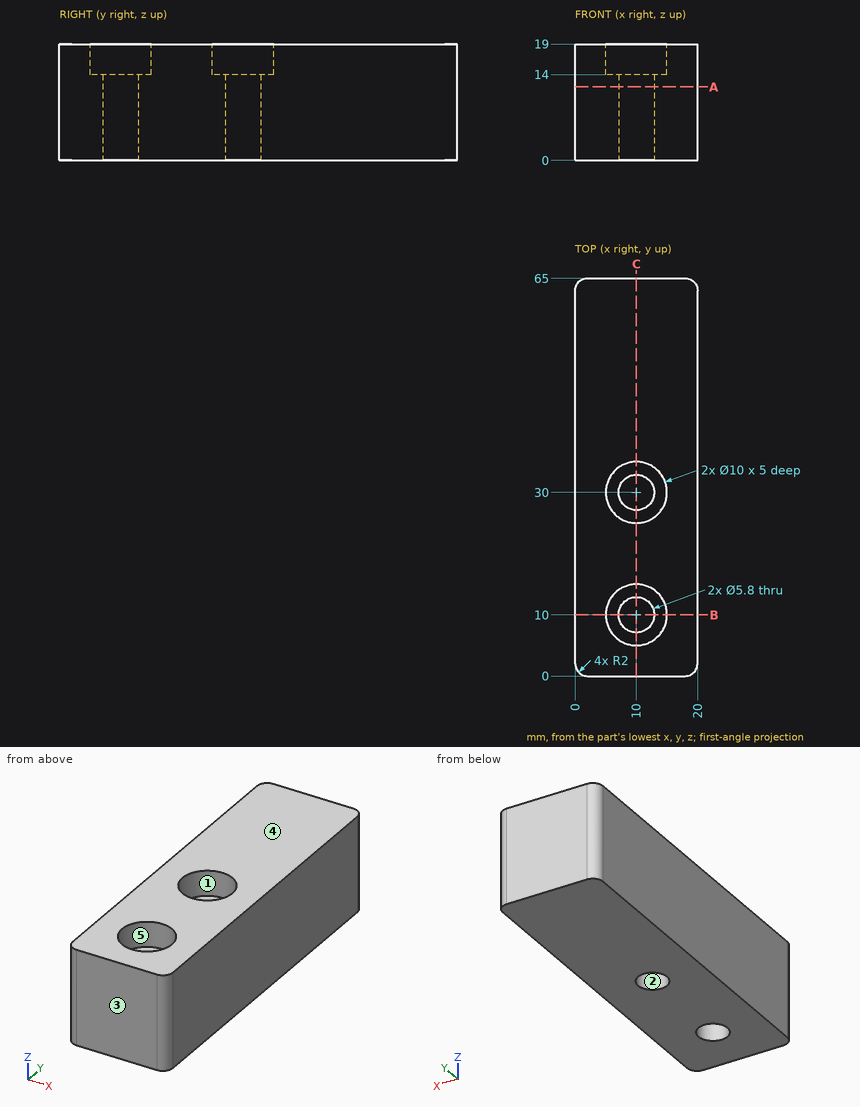
Input: dimensioned drawing with shaded views. Units: mm. Origin: part minimum x, y, z. A direction names the side the tool comes from. Round coordinates to 2 decimals unless told otherwise and drop trailing zeros. Write each loop counter-clockwise with the first axis right and the second up, starting at its lowest first coordinate (ties: lowest second). Pieces come first, ordered by that corner, then holes. Notation, with made-up numbers: (53, 46.5) - (85, 46.5) arc R13 cw to (85, 54.5) - close; hole circle Ø1 at (50, 51). An arc over 180 degrees is marked (long way). Write item = value, one per line.
(1) Access query for the marked faces 1 and 2. Directions: +Z, -Z, +X, -X, +Y, -Y. A direction counts if a zero-diameter tool reaches every point of the face in a straight line with its end or side. Return the directions, or none.
Geometry check:
face_1 = +Z
face_2 = +Z, -Z
(2) Material intervals for probe 1 along Y at (x, z) = (10, 5.5); probe 2 along Y at (x, z) = (8.5, 7.5); probe 3 along X at (y, z) = (29.5, 14.75), sorted ascending.
Geometry check:
probe_1 = 0 to 7.1, 12.9 to 27.1, 32.9 to 65
probe_2 = 0 to 7.52, 12.48 to 27.52, 32.48 to 65
probe_3 = 0 to 5.03, 14.97 to 20
(3) Section query A-A on z = 12. Output: boundary loops of the cut face in (x, y), then the cut area to 3 significant figures.
Geometry check:
outline = (0, 2) arc R2 ccw to (2, 0) - (18, 0) arc R2 ccw to (20, 2) - (20, 63) arc R2 ccw to (18, 65) - (2, 65) arc R2 ccw to (0, 63) - close; hole circle Ø5.8 at (10, 10); hole circle Ø5.8 at (10, 30)
area = 1,240 mm^2
(4) Contact query for a flat-ended pin moving along its axis: pin 1 Ø3 at (x, y) = (8, 10) entering from +Z. Output: stop coordinate, or through.
Geometry check:
pin_1 = 14
(5) Pull-direction query (Y, two-part tool) for the marked faces 3, 4 and 5; classes: +Y half, -Y half, draft (parallel to the pull), parting line (faces both ways), or undercut.
Geometry check:
face_3 = -Y half
face_4 = draft
face_5 = undercut
(6) Section query C-C on x = 10. Output: boundary loops of the cut face in (y, z), then the cut area to 3 significant figures.
Geometry check:
outline = (0, 0) - (7.1, 0) - (7.1, 14) - (5, 14) - (5, 19) - (0, 19) - close; (12.9, 0) - (27.1, 0) - (27.1, 14) - (25, 14) - (25, 19) - (15, 19) - (15, 14) - (12.9, 14) - close; (32.9, 0) - (65, 0) - (65, 19) - (35, 19) - (35, 14) - (32.9, 14) - close
area = 973 mm^2
(7) Section query B-B on y = 10. Output: boundary loops of the cut face in (x, z), then the cut area to 3 significant figures.
Geometry check:
outline = (0, 0) - (7.1, 0) - (7.1, 14) - (5, 14) - (5, 19) - (0, 19) - close; (12.9, 0) - (20, 0) - (20, 19) - (15, 19) - (15, 14) - (12.9, 14) - close
area = 249 mm^2
